Job drawing, mm, ordinate dimensions from the low corner. One solid piece. A direction names the side the tool comes from. Give positions to 0.01 mm unless a question says otherwise; leave off trailing zeros. Loops run counter-clockwise (first coordinate to the right, second up) from the corner with the lowest first, then second, coordinate; pieces in that order, holes last.
Item 1: Saw through at C-C on y = 7. Give the cut face in (x, z), plus the area to 3 significant figures.
Item 2: Saw through at A-A on z = 3.75. Give the cut face in (x, y), plus the area to 3 significant figures.
Item 3: Drop flat-ended pins along their axis: P1, Ø6, axis at x = 11, y = 8.5, coming from the -Z side; P2, Ø1.6, axis at x = 3, y = 9.5, coming from the -Z side; P3, Ø2, axis at x = 12, y = 3.5, coming from the +Z side; P4, Ø2.5, axis at x = 2.5, y = 8, coming from the -Z side. Give the stop position or say it passes through.
Item 4: Saw through at B-B on x = 9. Give the cut face in (y, z), plus the area to 3 significant figures.
Item 5: Saw through at D-D on z = 1.6. Give the cut face in (x, y).
Item 6: Mould opens along Y. For the marked faces 1, 2 and 3 say: released by +Y, released by -Y, zero draft, split by the parting line, or undercut.
Item 7: Which spindle directions (+Z, -Z, +X, -X, +Y, -Y) get a long thin tool onto all of the face, cutting with end or side? Do the marked faces 4, 5, 6 and 7. Say none if no direction does.
Item 8: Probe probe 1 along Y at (x, z) = (9, 2.05); probe 2 along Y at (x, z) = (2.5, 1.85); probe 3 along X at (y, z) = (4.75, 2.75). List the from-to ranges inside material, lowest first.
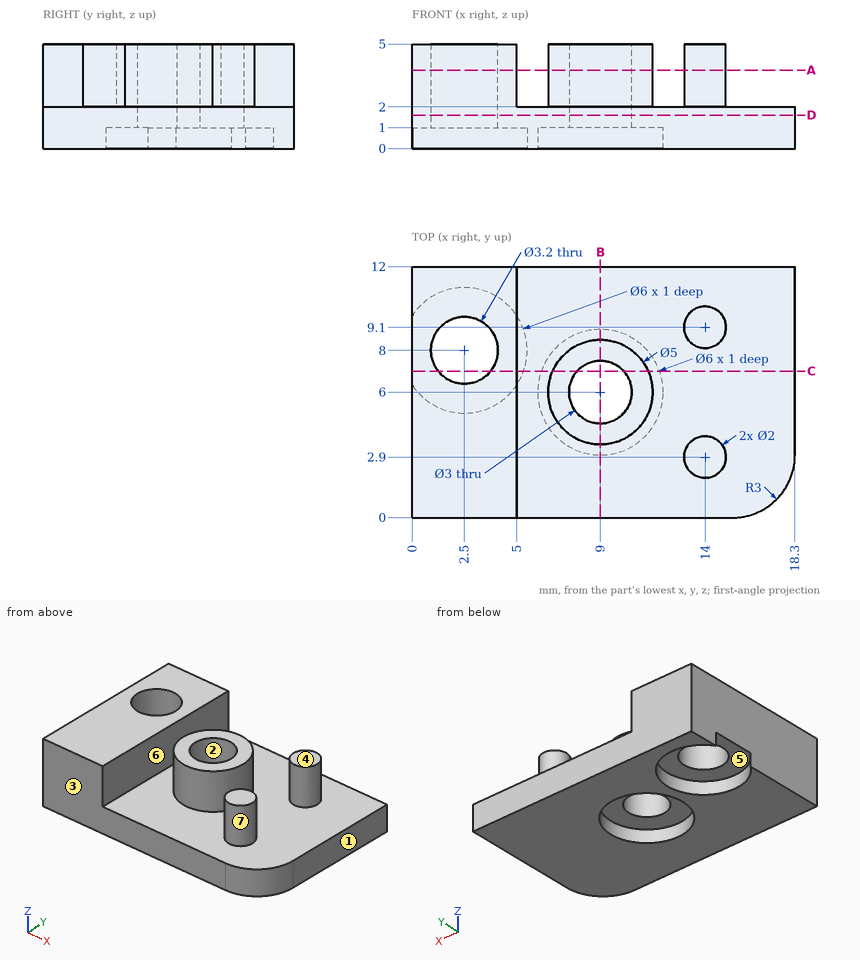
Results below:
1. outline: (0, 1) - (1.25, 1) - (1.25, 5) - (0, 5) - close; (3.75, 1) - (5.33, 1) - (5.33, 0) - (6.17, 0) - (6.17, 1) - (7.88, 1) - (7.88, 5) - (6.71, 5) - (6.71, 2) - (5, 2) - (5, 5) - (3.75, 5) - close; (10.12, 1) - (11.83, 1) - (11.83, 0) - (18.3, 0) - (18.3, 2) - (11.29, 2) - (11.29, 5) - (10.12, 5) - close
1. area: 35.4 mm2
2. outline: (0, 0) - (5, 0) - (5, 12) - (0, 12) - close; circle Ø5 at (9, 6); circle Ø2 at (14, 2.9); circle Ø2 at (14, 9.1); hole circle Ø3.2 at (2.5, 8); hole circle Ø3 at (9, 6)
2. area: 70.8 mm2
3. P1: stops at z = 0
3. P2: stops at z = 1
3. P3: stops at z = 2
3. P4: passes through
4. outline: (0, 0) - (3, 0) - (3, 1) - (4.5, 1) - (4.5, 5) - (3.5, 5) - (3.5, 2) - (0, 2) - close; (7.5, 1) - (9, 1) - (9, 0) - (12, 0) - (12, 2) - (8.5, 2) - (8.5, 5) - (7.5, 5) - close
4. area: 21.0 mm2
5. outline: (0, 0) - (15.3, 0) arc R3 ccw to (18.3, 3) - (18.3, 12) - (0, 12) - close; hole circle Ø3.2 at (2.5, 8); hole circle Ø3 at (9, 6)
6. face 1: zero draft
6. face 2: undercut
6. face 3: released by -Y
7. face 4: +Z, +X, -X, +Y, -Y
7. face 5: -Z
7. face 6: +Z, +Y, -Y
7. face 7: +Z
8. probe 1: y = 3.5 to 4.5, 7.5 to 8.5
8. probe 2: y = 0 to 6.4, 9.6 to 12
8. probe 3: x = 0 to 5, 6.83 to 8.17, 9.83 to 11.17
